Design review of the part built by this model. Coordinates are the model's own, in mm. A direction names the side the tool comes from. Round coordinates to 2 decimals unless told otherwise and drop trailing zeros. Write each loop counter-clockwise with the first axis right and the second up, starting at its lowest first coordinate (ties: lowest second). Pieces come first, ordered by that corner, then holes. Notation, with made-up numbers: (85.25, -12.75) -> (126.25, -12.75) arc R28 cw to (126.25, 23.25) -> close; hole circle Ø2 at (-40, 15). An arc over 180 degrees is marked (long way). Write item = value, one per line. Start each with the question number.
Item 1: Add section B-B, the plane x = -6.25. State the section outline as (y, z) points, then the cut area to 3 significant figures.
Item 2: Add section C-C, the plane y = 21. State the section outline as (x, z) points.
Item 3: Mouldability with a two-part tool opening along Y and no side actions: class faces 1 (the flat face through (-12.69, 56.29, -1.49)), 2 (the flat face through (-11.5, 44, -2)), 3 (the cylindrical face through (-15.95, 59.17, 1.49)) as released by +Y, released by -Y, zero draft, split by the parting line, or undercut.
Item 4: For pin 1 Ø1 at (x, z) = (-8.5, 0) entering from +Y; pin 2 Ø1.8 at (x, y) = (-15.5, 50) entering from +Z; pin 3 Ø3 at (x, z) = (0.5, 3) entering from +Y; pin 4 Ø2.5 at (x, y) = (-10, 50) entering from +Z, all flat-tipped, find the tip position at first contact; note any pin that passes through.
Item 5: To check wall thickness, follow L1, parallel to Y at x = -10, z = 2.45; L2, parallel to Z at x = -14.75, y = 48; L3, parallel to Z at x = 0, y = 15.5. State the ranges of each line that lie inside material, in increasing order.
Item 6: Machinability: for faces 4 (the flat face through (-15, 55, -0.75)), 5 (the flat face through (-11, 49, 1)), 6 (the flat face through (-15, 55, -2.25)), 7 (the flat face through (3.3, 30, 4.1)), which of the approach directions +Z, -Z, +X, -X, +Y, -Y give a long, thin tool a straight path to every point of the face, cutting with its end or side? Answer none if there is none.
Item 7: Add section A-A, the plane z = 0. State the section outline as (x, y) points, then the cut area to 3 significant figures.
Autodesk Inventor part; units mm, degrees
ref_plane "Work Plane1" through (0, 0, 0.75) normal (0, 0, 1) x (1, 0, 0)
ref_plane "YZ Plane" through (0, 0, 0) normal (1, 0, 0) x (0, 1, 0)
ref_plane "XZ Plane" through (0, 0, 0) normal (0, 1, 0) x (-1, 0, 0)
sketch "Sketch1" plane through (0, 0, 0) normal (0, 1, 0) x (-1, 0, 0)
  circle A0 centre (0, 0) radius 5
  circle A1 centre (0, 0) radius 5.5
  dimension "d0" = 10
  dimension "d1" = 11
extrude "Extrusion1" add sketch "Sketch1" along normal blind 35
sketch "Sketch2" plane through (0, 0, 0) normal (0, 0, 1) x (1, 0, 0)
  point P0 (0, 0)
sketch "Sketch3" plane through (0, 0, 0) normal (0, 0, 1) x (1, 0, 0)
  line L0 (0, 0) -> (-10, 0)
  line L1 (-5.5, 0) -> (5.5, 0)
  circle A0 centre (-10, 50) radius 1
  line L2 (-5.5495, 50) -> (-5.5, 50)
  line L3 (-5.5, 50) -> (-5.5, 35)
  line L4 (5.5, 35) -> (-5.5, 35)
  line L5 (-14.5, 50) -> (-14.5, 0)
  line L6 (-14.5, 0) -> (-10, 0)
  circle A1 centre (-10, 50) radius 4.5
  line L7 (-10, 45.5) -> (-5.5, 45.5)
  line L8 (-14.5, 45.5) -> (-10, 45.5)
  line L9 (-5.5, 0) -> (-5.5, 50)
  line L10 (-5.5, 0) -> (-5.5, 45.5)
  line L11 (5, 0) -> (-5, 0)
  line L12 (-5.5, 0) -> (-5.5, 45.5)
  line L13 (-10, 0) -> (-5, 0)
  line L14 (-5.5, 45.5) -> (-5, 0)
  line L15 (-10, 0) -> (-10, 45.5)
  line L16 (-10, 45.5) -> (-5.5, 45.5)
  line L17 (-9, 50) -> (-10, 50)
  line L18 (-11, 50) -> (-14.5, 50)
  line L19 (-10, 0) -> (-10, 45.5)
  line L20 (-10, 49) -> (-10, 50)
  circle A2 centre (-10, 50) radius 4.5
  line L21 (-14.5, 45.5) -> (-14.5, 50)
  line L22 (-14.5, 45.5) -> (-5.5, 45.5)
  line L23 (-5.5, 45.5) -> (-5.5, 50)
  line L24 (-10, 50) -> (0, 50) construction
  line L25 (-10, 50) -> (-10.5736, 50.8192)
  circle A3 centre (-15.7358, 58.1915) radius 1
  circle A4 centre (-15.7358, 58.1915) radius 2.5
  point P0 (12.8857, 32.907)
  dimension "d4" = 10
  dimension "d5" = 50
  dimension "d7" = 2
  dimension "d8" = 9
  dimension "d19" = 2
  dimension "d20" = 5
extrude "Extrusion2" add sketch "Sketch3" along normal mid plane 2 contours L0 L9 L4 L14 | L0 L15 L7 L3 L9 | L4 L3 L14 | L6 L5 L8 L15
sketch "Sketch4" plane through (0, 0, 1) normal (0, 0, 1) x (1, 0, 0)
  circle A0 centre (-10, 50) radius 4.5
  line L0 (-14.5, 50) -> (-14.5, 0)
  line L1 (-5.5, 50) -> (-5.5, 35)
  line L2 (-5.5, 45.5) -> (-14.5, 45.5)
  arc A1 (-14.5, 50) -> (-10, 45.5) centre (-10, 50) ccw
  line L3 (-10, 45.5) -> (-14.5, 45.5)
  line L4 (-14.5, 45.5) -> (-14.5, 50)
  point P0 (0, 0)
extrude "Extrusion3" add sketch "Sketch4" along normal blind 2 contours A0 L2 L0
sketch "Sketch5" plane through (0, 0, 1) normal (0, 0, 1) x (1, 0, 0)
  line L0 (-5.3846, 35) -> (-5.5, 45.5)
  line L1 (-5.4396, 40) -> (-14.5, 40)
  line L2 (-14.5, 45.5) -> (-14.5, 0)
  point P0 (0, 0)
sketch "Sketch6" plane through (-14.5, 45.5, 1) normal (-1, 0, 0) x (0, 0, 1)
  line L0 (2, 0) -> (0, -5.25)
  line L1 (0, -10.5) -> (0, 0)
  line L2 (2, 0) -> (0, 0)
  line L3 (0, 0) -> (0, -5.25)
  point P0 (-1, -45.5)
extrude "Extrusion4" add sketch "Sketch6" against normal blind 3
sketch "Sketch7" plane through (0, 0, 3) normal (0, 0, 1) x (1, 0, 0)
  circle A0 centre (-10, 50) radius 4.5
  circle A1 centre (-10, 50) radius 1
  point P0 (0, 0)
extrude "Extrusion5" add sketch "Sketch7" against normal blind 2
mirror "Mirror1" about plane through (0, 0, 0) normal (0, 0, 1) of "Extrusion4", "Extrusion3", "Extrusion5"
ref_plane "Work Plane1" through (0, 0, 0.75) normal (0, 0, 1) x (1, 0, 0)
sketch "Sketch8" plane through (0, 0, 0.75) normal (0, 0, 1) x (1, 0, 0)
  circle A0 centre (-15.7358, 58.1915) radius 2.5
  circle A1 centre (-15.7358, 58.1915) radius 1
  line L0 (-14.5, 45.5) -> (-18.1282, 57.4661)
  line L1 (-13.3433, 58.9169) -> (-12.1116, 53.9738)
  arc A2 (-10, 45.5) -> (-14.5, 50) centre (-10, 50) ccw
  arc A3 (-12.1116, 53.9738) -> (-14.5, 50) centre (-10, 50) ccw
  line L2 (-14.5, 45.5) -> (-14.5, 50)
  line L3 (-14.5, 50) -> (-14.5, 45.5)
  point P0 (0, 0)
extrude "Extrusion6" add sketch "Sketch8" along normal blind 1.5
mirror "Mirror2" about plane through (0, 0, 0) normal (0, 0, 1) of "Extrusion6"
sketch "Sketch9" plane through (0, 0, 0) normal (0, 0, -1) x (1, 0, 0)
  point P0 (0, 0)
sketch "Sketch10" plane through (0, 35, 0) normal (0, 1, 0) x (1, 0, 0)
  line L0 (6.5, -1) -> (4.5, -1)
  line L1 (4.5, -1) -> (4.5, 1)
  line L2 (4.5, 1) -> (6.5, 1)
  line L3 (6.5, 1) -> (6.5, -1)
  arc A0 (-5.4083, -1) -> (-5.4083, 1) centre (0, 0) ccw
  line L4 (6.5, -1) -> (4.5, 1) construction
  line L5 (4.5, -1) -> (6.5, 1) construction
  point P0 (5.5, 0)
  dimension "d24" = 2
  dimension "d25" = 2
extrude "Extrusion7" cut sketch "Sketch10" against normal blind 10
sketch "Sketch11" plane through (0, 35, 0) normal (0, 1, 0) x (1, 0, 0)
  line L0 (0, 5.5536) -> (9.1038, 5.5536)
  line L1 (9.1038, 5.5536) -> (9.1038, -5.5536)
  line L2 (9.1038, -5.5536) -> (0, -5.5536)
  line L3 (0, -5.5536) -> (0, 5.5536)
  point P0 (0, 0)
extrude "Extrusion8" cut sketch "Sketch11" against normal blind 5
ref_plane "Work Plane2" through (0, 0, 0) normal (0, 0, 1) x (1, 0, 0)
properties part number "Base_Cylinder_1"
Result set:
q1.outline = (0, -1) -> (45.5, -1) -> (45.5, 1) -> (0, 1) -> close; (47.51, -3) -> (52.49, -3) -> (52.49, -1) -> (47.51, -1) -> close; (47.51, 1) -> (52.49, 1) -> (52.49, 3) -> (47.51, 3) -> close
q1.area = 111 mm²
q2.outline = (-14.5, -1) -> (-5.41, -1) arc R5.5 ccw (long way) to (-5.41, 1) -> (-14.5, 1) -> close; hole circle Ø10 at (0, 0)
q3.face_1 = released by +Y
q3.face_2 = zero draft
q3.face_3 = undercut
q4.pin_1 = 45.5
q4.pin_2 = 2.25
q4.pin_3 = through
q4.pin_4 = 3
q5.L1 = 45.5 to 49, 51 to 54.5
q5.L2 = -2.25 to -0.75, 0.75 to 2.25
q5.L3 = -5.5 to -5, 5 to 5.5
q6.face_4 = +X, -X, +Y
q6.face_5 = +X
q6.face_6 = -Z, -X, +Y
q6.face_7 = +Z, -Z, +X, +Y
q7.outline = (-14.5, 0) -> (-5, 0) -> (-5, 35) -> (-5.38, 35) -> (-5.5, 45.5) -> (-14.5, 45.5) -> close; (5, 0) -> (5.5, 0) -> (5.5, 25) -> (5, 25) -> close
q7.area = 440 mm²
